Read the model definition and answer for the solid it produces. Units are mm, in the model's axes. A direction names the side the tool comes from. Coordinates: 2 decimals unless noted, no trailing zeros. Write each loop counter-clockwise with the first axis right and the second up, starting at its lowest first coordinate (ties: lowest second). Pieces come first, ordered by that corner, then holes. Notation, with made-up numbers: (35.5, 24.25) -> (52.5, 24.25) arc R11 ccw to (52.5, 44.25) -> close; hole circle Ø11 at (-28, 4). An arc over 180 degrees is marked (long way). Answer in a Markdown table with one row per item. Add a question column.
Item 1: Section B-B on x = 136.5 is taken. Count the separate pieces of the cut face and the enclosed holes in it, then the cut area to 3 significant figures.
Item 2: Given pin 1 Ø12 at (x, y) = (146, 180.5) entering from +Z; pin 2 Ø2 at (y, z) = (34, -77.5) entering from +X; pin 3 Ø2 at (x, z) = (84, -113.5) entering from -Y; pin 4 Ø0.9 at (y, z) = (61, -416.5) entering from +X, each flat-ended and moving along its own axis, determine where each tip first touches the part or whether it passes through.
Item 3: Section A-A on z = -71.12 is taken. Write down the section's boundary in (x, y) (3 decimals).
Item 4: Which of the six approach directions +Z, -Z, +X, -X, +Y, -Y give full straight-line access (tool end or side, diameter ignored) to faces 4 (the face through (74, 281.94, -215)), 5 (the face through (-2.54, 81, -215)), 6 (the face through (95.25, 224, -14)), 7 (the face through (106.105, 222.702, -316.115)), 8 (the face through (145, 224, -63.5))?
Item 5: For a pull along X with two mould halves and no side action, classify faces 1 (the face through (-19.05, 140, -215)), 2 (the face through (102.77, 224.34, -220.21)), 3 (the face through (-9, -5.08, -211)) as +X half, -X half, draft (parallel to the pull), parting line (faces both ways), or undercut.
Item 6: Straight lines are drawn through the part: line 1 (Z direction, x = 82, y = 237); line 2 (X direction, y = 238.5, z = -165.1) (3 decimals); line 3 (Z direction, x = 11, y = 142.5). For each, find the intervals that lie inside material, in ascending order. Write a range as from..to.
Item 7: Section C-C on y = 76.2 is taken. Write down the section's boundary in (x, z) (3 decimals), then the cut area to 3 significant figures.
Item 8: Section D-D on x = 16 is taken. Write down the section's boundary in (y, z), then the cut area to 3 significant figures.
Autodesk Inventor part; units mm, degrees
ref_plane "Work Plane1" through (82.55, 89.535, -212.09) normal (0, 0, 1) x (1, 0, 0)
ref_plane "YZ Plane" through (0, 0, 0) normal (1, 0, 0) x (0, 1, 0)
ref_plane "XZ Plane" through (0, 0, 0) normal (0, 1, 0) x (-1, 0, 0)
sketch "Sketch1" plane through (0, 0, 0) normal (1, 0, 0) x (0, 1, 0)
  line L0 (0, 0) -> (228.6, 0)
  line L1 (228.6, 0) -> (228.6, -424.18)
  line L2 (228.6, -424.18) -> (0, -424.18)
  line L3 (0, -424.18) -> (0, 0)
  point P0 (0, 0)
  dimension "d0" = 424.18
  dimension "d1" = 228.6
extrude "Extrusion1" add sketch "Sketch1" along normal blind 165.1
sketch "Sketch2" plane through (165.1, 0, 0) normal (1, 0, 0) x (0, 0, -1)
  line L0 (0, 0) -> (424.18, 0) construction
  line L1 (12.7, 0) -> (411.48, 0)
  line L2 (411.48, 0) -> (411.48, 165.1)
  line L3 (411.48, 165.1) -> (12.7, 165.1)
  line L4 (12.7, 165.1) -> (12.7, 0)
  line L5 (0, 228.6) -> (0, 0) construction
  line L6 (424.18, 0) -> (424.18, 228.6) construction
  dimension "d4" = 398.78
  dimension "d5" = 165.1
  dimension "d6" = 12.7
  dimension "d7" = 12.7
extrude "Extrusion2" cut sketch "Sketch2" against normal blind 148.59
sketch "Sketch3" plane through (0, 0, 0) normal (0, 0, 1) x (1, 0, 0)
  line L0 (165.1, 228.6) -> (165.1, 0)
  line L1 (165.1, 89.535) -> (82.55, 89.535)
  line L2 (69.215, 89.535) -> (69.215, 62.865) construction
  line L3 (82.55, 62.865) -> (165.1, 62.865)
  line L4 (165.1, 62.865) -> (165.1, 89.535)
  line L5 (0, 0) -> (165.1, 0)
  arc A0 (82.55, 89.535) -> (82.55, 62.865) centre (82.55, 76.2) ccw
  dimension "d10" = 95.885
  dimension "d11" = 26.67
  dimension "d12" = 62.865
extrude "Extrusion3" cut sketch "Sketch3" against normal blind 457.2
sketch "Sketch4" plane through (0, 228.6, 0) normal (0, 1, 0) x (1, 0, 0)
  line L0 (165.1, 12.7) -> (165.1, 411.48) construction
  line L1 (165.1, 12.7) -> (16.51, 12.7) construction
  line L2 (16.51, 12.7) -> (16.51, 411.48) construction
  line L3 (165.1, 411.48) -> (16.51, 411.48) construction
  line L4 (0, 424.18) -> (165.1, 424.18) construction
  line L5 (0, 424.18) -> (165.1, 424.18) construction
  circle A0 centre (82.55, 353.06) radius 43.815
  line L6 (0, 0) -> (0, 424.18) construction
  circle A1 centre (82.55, 259.08) radius 43.815
  line L7 (0, 212.09) -> (165.1, 212.09) construction
  line L8 (165.1, 424.18) -> (165.1, 0) construction
  circle A2 centre (82.55, 71.12) radius 43.815
  circle A3 centre (82.55, 165.1) radius 43.815
  dimension "d15" = 87.63
  dimension "d16" = 82.55
  dimension "d17" = 58.42
  dimension "d18" = 87.63
  dimension "d19" = 93.98
  dimension "d20" = 82.55
extrude "Extrusion4" cut sketch "Sketch4" against normal blind 76.2
sketch "Sketch5" plane through (0, 228.6, 0) normal (0, 1, 0) x (1, 0, 0)
  circle A0 centre (82.55, 165.1) radius 43.815
  circle A1 centre (82.55, 353.06) radius 43.815
  circle A2 centre (82.55, 259.08) radius 43.815
  circle A3 centre (82.55, 71.12) radius 43.815
  line L0 (0, 0) -> (0, 424.18)
  line L1 (0, 0) -> (165.1, 0)
  line L2 (165.1, 424.18) -> (165.1, 0)
  line L3 (0, 424.18) -> (165.1, 424.18)
  point P0 (0, 0)
extrude "Extrusion5" add sketch "Sketch5" along normal blind 53.34
sketch "Sketch7" plane through (0, 0, 0) normal (-1, 0, 0) x (0, 0, 1)
  line L0 (0, 0) -> (0, 281.94)
  line L1 (-424.18, 281.94) -> (0, 281.94)
  line L2 (-424.18, 281.94) -> (-424.18, 0)
  line L3 (-424.18, 0) -> (0, 0)
  point P0 (0, 0)
extrude "Extrusion6" add sketch "Sketch7" along normal blind 19.05
sketch "Sketch8" plane through (16.51, 0, 0) normal (1, 0, 0) x (0, 0, -1)
  line L0 (411.48, 0) -> (12.7, 0)
  line L1 (411.48, 165.1) -> (411.48, 0)
  line L2 (12.7, 165.1) -> (411.48, 165.1)
  line L3 (12.7, 0) -> (12.7, 165.1)
  point P0 (0, 0)
extrude "Extrusion7" cut sketch "Sketch8" against normal blind 19.05
sketch "Sketch12" plane through (165.1, 0, 0) normal (1, 0, 0) x (0, 0, -1)
  line L0 (0, 89.535) -> (12.7, 89.535) construction
  line L1 (3.302, 89.535) -> (9.398, 89.535)
  line L2 (9.398, 89.535) -> (9.398, 92.583)
  line L3 (9.398, 92.583) -> (3.302, 92.583)
  line L4 (3.302, 92.583) -> (3.302, 89.535)
  line L5 (0, 89.535) -> (0, 281.94) construction
  line L6 (12.7, 89.535) -> (12.7, 62.865) construction
  line L7 (0, 89.535) -> (12.7, 89.535) construction
  line L8 (0, 62.865) -> (0, 89.535) construction
  line L9 (0, 62.865) -> (12.7, 62.865) construction
  line L10 (0, 62.865) -> (0, 89.535) construction
  line L11 (0, 76.2) -> (12.7, 76.2) construction
  line L12 (3.302, 62.865) -> (9.398, 62.865)
  line L13 (9.398, 62.865) -> (9.398, 59.817)
  line L14 (9.398, 59.817) -> (3.302, 59.817)
  line L15 (3.302, 59.817) -> (3.302, 62.865)
  point P0 (0, 0)
  dimension "d44" = 6.096
  dimension "d45" = 3.048
  dimension "d46" = 3.302
extrude "Extrusion11" cut sketch "Sketch12" against normal blind 82.55
sketch "Sketch13" plane through (-19.05, 0, 0) normal (0, -1, 0) x (1, 0, 0)
  line L0 (16.51, -12.7) -> (184.15, -12.7)
  line L1 (184.15, 0) -> (184.15, -12.7)
  line L2 (0, 0) -> (184.15, 0)
  line L3 (0, -424.18) -> (0, 0)
  line L4 (184.15, -424.18) -> (0, -424.18)
  line L5 (184.15, -411.48) -> (184.15, -424.18)
  line L6 (184.15, -411.48) -> (16.51, -411.48)
  line L7 (16.51, -411.48) -> (16.51, -12.7)
  point P0 (19.05, 0)
extrude "Extrusion12" add sketch "Sketch13" along normal blind 5.08
ref_plane "Work Plane1" through (82.55, 89.535, -212.09) normal (0, 0, 1) x (1, 0, 0)
mirror "Mirror1" about plane through (82.55, 89.535, -212.09) normal (0, 0, 1) of "Extrusion11"
sketch "Sketch21" plane through (0, 281.94, 0) normal (0, 1, 0) x (1, 0, 0)
  line L0 (165.1, 0) -> (95.25, 0)
  line L1 (95.25, 0) -> (95.25, 63.5)
  line L2 (95.25, 63.5) -> (165.1, 63.5)
  line L3 (165.1, 63.5) -> (165.1, 0)
  point P0 (0, 0)
  point P1 (165.1, 0)
  dimension "d70" = 63.5
  dimension "d71" = 69.85
extrude "Extrusion18" cut sketch "Sketch21" against normal blind 116.84
sketch "Sketch9" plane through (0, 281.94, 0) normal (0, 1, 0) x (1, 0, 0)
  line L0 (146.05, 19.05) -> (146.05, 405.13)
  line L1 (0, 405.13) -> (0, 19.05)
  line L2 (165.1, 424.18) -> (-19.05, 424.18) construction
  line L3 (-19.05, 0) -> (-19.05, 424.18) construction
  line L4 (165.1, 0) -> (165.1, 424.18) construction
  line L5 (165.1, 0) -> (-19.05, 0) construction
  circle A0 centre (82.55, 71.12) radius 43.815 construction
  circle A1 centre (82.55, 259.08) radius 43.815 construction
  circle A2 centre (82.55, 353.06) radius 43.815 construction
  circle A3 centre (82.55, 165.1) radius 43.815 construction
  line L6 (165.1, 0) -> (-19.05, 0) construction
  line L7 (165.1, 0) -> (165.1, 424.18) construction
  line L8 (165.1, 424.18) -> (-19.05, 424.18) construction
  line L9 (-19.05, 0) -> (-19.05, 424.18) construction
  line L10 (146.05, 405.13) -> (117.7739, 405.13)
  line L11 (47.3261, 405.13) -> (0, 405.13)
  arc A4 (47.3261, 405.13) -> (40.7894, 306.07) centre (82.55, 353.06) ccw
  arc A5 (124.3106, 306.07) -> (117.7739, 405.13) centre (82.55, 353.06) ccw
  arc A6 (40.7894, 306.07) -> (40.7894, 212.09) centre (82.55, 259.08) ccw
  arc A7 (124.3106, 212.09) -> (107.2668, 316.8822) centre (82.55, 259.08) ccw
  arc A8 (40.7894, 212.09) -> (40.7894, 118.11) centre (82.55, 165.1) ccw
  arc A9 (124.3106, 118.11) -> (124.3106, 212.09) centre (82.55, 165.1) ccw
  line L12 (0, 19.05) -> (47.3261, 19.05)
  line L13 (117.7739, 19.05) -> (146.05, 19.05)
  arc A10 (40.7894, 118.11) -> (47.3261, 19.05) centre (82.55, 71.12) ccw
  arc A11 (117.7739, 19.05) -> (124.3106, 118.11) centre (82.55, 71.12) ccw
  point P0 (0, 0)
  dimension "d30" = 19.05
  dimension "d31" = 19.05
sketch "Sketch10" plane through (0, 281.94, -19.05) normal (1, 0, 0) x (0, 0, -1)
  line L0 (405.13, 0) -> (405.13, -281.94)
  line L1 (-19.05, 0) -> (405.13, 0)
  line L2 (405.13, -101.6) -> (-19.05, -101.6)
  line L3 (-19.05, -101.6) -> (-19.05, 0)
  line L4 (-19.05, 0) -> (405.13, 0)
  line L5 (405.13, 0) -> (405.13, -101.6)
  line L6 (0, 0) -> (386.08, 0)
  line L7 (0, 0) -> (0, -101.6)
  line L8 (0, -101.6) -> (386.08, -101.6)
  line L9 (386.08, 0) -> (386.08, -101.6)
  point P0 (-19.05, -281.94)
  dimension "d39" = 0
sketch "Sketch11" plane through (0, 281.94, 0) normal (0, 1, 0) x (1, 0, 0)
  circle A0 centre (82.55, 71.12) radius 43.815 construction
  line L0 (19.05, 19.05) -> (19.05, 0)
  line L1 (19.05, 0) -> (47.3261, 0)
  line L2 (47.3261, 0) -> (47.3261, 19.05)
  line L3 (47.3261, 19.05) -> (19.05, 19.05)
  line L4 (19.05, 19.05) -> (19.05, 0)
  line L5 (165.1, 424.18) -> (19.05, 424.18)
  line L6 (47.3261, 405.13) -> (19.05, 405.13)
  line L7 (19.05, 405.13) -> (19.05, 424.18)
  line L8 (19.05, 424.18) -> (47.3261, 424.18)
  line L9 (47.3261, 424.18) -> (47.3261, 405.13)
  point P0 (0, 0)
properties part number "Engine Block"
Results below:
| question | item | result |
|---|---|---|
| 1 | separate pieces | 4 |
| 1 | enclosed holes | 0 |
| 1 | area | 45,700 mm2 |
| 2 | pin 1 | stops at z = -63.5 |
| 2 | pin 2 | stops at x = -2.54 |
| 2 | pin 3 | passes through |
| 2 | pin 4 | stops at x = 82.55 |
| 3 | outline | (-19.05, -5.08) -> (-2.54, -5.08) -> (-2.54, 165.1) -> (38.735, 165.1) -> (38.735, 281.94) -> (-19.05, 281.94) -> close; (126.365, 165.1) -> (165.1, 165.1) -> (165.1, 281.94) -> (126.365, 281.94) -> close |
| 4 | face 4 | +Z, -Z, +X, -X, +Y |
| 4 | face 5 | +X, -Y |
| 4 | face 6 | +Z, +X, +Y |
| 4 | face 7 | +Y, -Y |
| 4 | face 8 | +Z, +X, +Y, -Y |
| 5 | face 1 | -X half |
| 5 | face 2 | undercut |
| 5 | face 3 | draft |
| 6 | line 1 | z = -424.18..-396.87, -309.25..-302.89, -215.27..-208.91, -121.29..-114.93, -27.31..0 |
| 6 | line 2 | x = -19.05..38.735, 126.365..165.1 |
| 6 | line 3 | z = -424.18..-411.48, -12.7..0 |
| 7 | outline | (-19.05, -424.18) -> (69.215, -424.18) -> (69.215, -411.48) -> (-2.54, -411.48) -> (-2.54, -12.7) -> (69.215, -12.7) -> (69.215, 0) -> (-19.05, 0) -> close |
| 7 | area | 8,830 mm2 |
| 8 | outline | (-5.08, -424.18) -> (281.94, -424.18) -> (281.94, 0) -> (-5.08, 0) -> (-5.08, -12.7) -> (165.1, -12.7) -> (165.1, -411.48) -> (-5.08, -411.48) -> close |
| 8 | area | 53,900 mm2 |
